Build history of the part. All positions in model axes, mm. A direction names the side the tool comes from. Give positions to 0.01 mm unless a question says otherwise; leave off trailing zeros. Write each loop counter-clockwise with the first axis right and the second up, starting at its lowest first coordinate (ties: lowest second). Pieces come first, ordered by that corner, then holes.
from build123d import *

# Parameters (mm, degrees)
SKETCH1_R           = 20
BOSS_EXTRUDE2_DEPTH = 20
SKETCH8_R           = 25
CUT_EXTRUDE6_DEPTH  = 5


with BuildPart() as part:
    # Sketch1 → Boss-Extrude2 (new body)
    with BuildSketch(Plane.XY):
        with BuildLine():
            Line((474.74714713, 99.423872527), (-150.25285287, 99.423872527))
            ThreePointArc((-150.25285287, 99.423872527), (-250.25285287, -0.576127473), (-150.25285287, -100.576127473))
            Line((-150.25285287, -100.576127473), (474.74714713, -100.576127473))
            ThreePointArc((474.74714713, -100.576127473), (574.74714713, -0.576127473), (474.74714713, 99.423872527))
        make_face()
        with Locations((-150.25285287, -0.576127473)):
            Circle(SKETCH1_R, mode=Mode.SUBTRACT)
        with Locations(Location((474.74714713, -0.576127473, 0), (0, 0, 180))):
            Circle(SKETCH1_R, mode=Mode.SUBTRACT)
    extrude(amount=BOSS_EXTRUDE2_DEPTH)

    # Sketch8 → Cut-Extrude6 (cut)
    with BuildSketch(Plane.XY):
        with BuildLine():
            Line((-150.25285287, -95.576127473), (474.74714713, -95.576127473))
            ThreePointArc((474.74714713, -95.576127473), (569.74714713, -0.576127473), (474.74714713, 94.423872527))
            Line((474.74714713, 94.423872527), (-150.25285287, 94.423872527))
            ThreePointArc((-150.25285287, 94.423872527), (-245.25285287, -0.576127473), (-150.25285287, -95.576127473))
        make_face()
        with Locations((-150.25285287, -0.576127473)):
            Circle(SKETCH8_R, mode=Mode.SUBTRACT)
    extrude(amount=CUT_EXTRUDE6_DEPTH, mode=Mode.SUBTRACT)


solid = part.part
(1) Saw through at B-B, the plane z = 16. List the corners of the cut face in (x, y).
(2) Probe line 1 (X direction, y = 16.5, z = 17); line 2 (X direction, y = 8, z = 11.5); line 3 (Y direction, x = 245, z = 1.5). List the from-to ranges inside material, lowest first.
(3) Drop flat-ended pins along their axis: pin 1 (2 mm diameter, centred on y = 35, z = 4.5, fed in from -X); pin 2 (4 mm diameter, centred on y = 17, z = 15, fed in from +X); pin 3 (10 mm diameter, centred on x = -116, y = -2.5, fed in from -Z). Give the stop position or say it passes through.
(4) Saw through at A-A, the plane x = 165. List the corners of the cut face in (y, z).
(5) 3-axis set-ups, long thin cutter, end or side, ignore diameter. For faces 4 (the face through (156, 1, 20)), 5 (the face through (157, 1, 5)): which of +Z, -Z, +X, -X, +Y, -Y reach the whole face in a straight line?
(6) Saw through at C-C, the plane y = 78. List the corners of the cut face in (x, z), plus the area to 3 significant figures.
(7) Mould opens along Y. For faces 1 (the face through (494.728, -1.455, 12.395)), 2 (the face through (160, -96, 0)), 3 (the face through (167, 99.424, 10)) say: +Y half, -Y half, draft (parallel to the pull), parting line (faces both ways), or undercut.
Computed values:
1. outline: (-150.25, -100.58) - (474.75, -100.58) arc R100 ccw to (474.75, 99.42) - (-150.25, 99.42) arc R100 ccw to start; hole circle Ø40 at (-150.25, -0.58); hole circle Ø40 at (474.75, -0.58)
2. line 1: x = -248.78 to -160.66, -139.84 to 464.34, 485.16 to 573.28
2. line 2: x = -249.88 to -168.32, -132.18 to 456.68, 492.82 to 574.38
2. line 3: y = -100.58 to -95.58, 94.42 to 99.42
3. pin 1: stops at x = -244.09
3. pin 2: stops at x = 573.53
3. pin 3: stops at z = 5
4. outline: (-100.58, 0) - (-95.58, 0) - (-95.58, 5) - (94.42, 5) - (94.42, 0) - (99.42, 0) - (99.42, 20) - (-100.58, 20) - close
5. face 4: +Z, +X, -X, +Y, -Y
5. face 5: -Z
6. outline: (-212.11, 0) - (-203.65, 0) - (-203.65, 5) - (528.14, 5) - (528.14, 0) - (536.6, 0) - (536.6, 20) - (-212.11, 20) - close
6. area: 11,300 mm2
7. face 1: undercut
7. face 2: draft
7. face 3: +Y half
